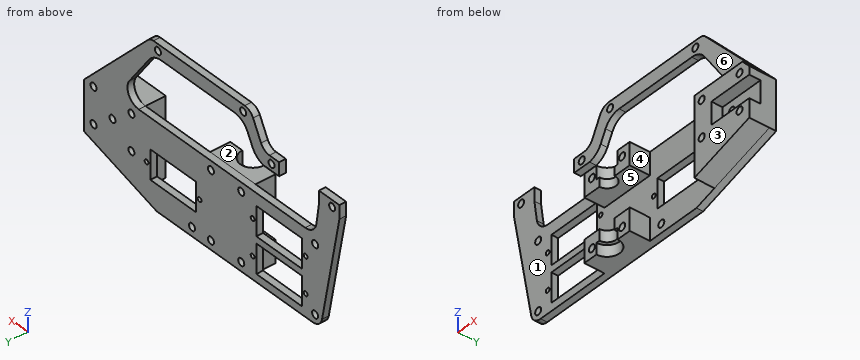
```python
from build123d import *

# Parameters (mm, degrees)
SKETCH_1_R          = 1.6
SKETCH_1_R_2        = 1
SKETCH_1_W          = 24
SKETCH_1_H          = 13
EXTRUDE_1_DEPTH     = 3
SKETCH_2_R          = 1.6
SKETCH_2_W          = 24
SKETCH_2_H          = 10
EXTRUDE_2_DEPTH     = 9
SKETCH_3_W          = 10
SKETCH_3_H          = 10
CUT_EXTRUDE_1_DEPTH = 20
SKETCH_4_R          = 4
CUT_EXTRUDE_2_DEPTH = 72.704206567
SKETCH_6_R          = 5.6
CUT_EXTRUDE_3_DEPTH = 5
SKETCH_7_R          = 5.6
CUT_EXTRUDE_4_DEPTH = 6
FILLET_5_R          = 5
FILLET_6_R          = 5
SKETCH_8_W          = 21
SKETCH_8_H          = 6
CUT_EXTRUDE_5_DEPTH = 13


with BuildPart() as part:
    # Эскиз1 → Бобышка-Вытянуть1 (new body)
    with BuildSketch(Plane(origin=(0, 0, 0), x_dir=(1, 0, 0), z_dir=(0, 1, 0))):
        with BuildLine():
            Line((-59.846473334, -34), (-49.887758312, 18))
            Line((-49.887758312, 18), (36.612736258, 18))
            Line((36.612736258, 18), (75.112241688, 5.920216985))
            Line((75.112241688, 5.920216985), (75.112241688, -16.079783015))
            Line((75.112241688, -16.079783015), (41.245672077, -52.430849732))
            ThreePointArc((41.245672077, -52.430849732), (39.914841322, -53.372078747), (38.318998701, -53.704206567))
            Line((38.318998701, -53.704206567), (-9.799827382, -53.704206567))
            ThreePointArc((-9.799827382, -53.704206567), (-12.412320205, -52.967407389), (-14.254860003, -50.974159066))
            Line((-14.254860003, -50.974159066), (-19.846473334, -40))
            Line((-19.846473334, -40), (-59.846473334, -40))
            Line((-59.846473334, -40), (-59.846473334, -34))
        make_face()
        with Locations((-8, 14)):
            Circle(SKETCH_1_R, mode=Mode.SUBTRACT)
        with Locations((8, 14)):
            Circle(SKETCH_1_R, mode=Mode.SUBTRACT)
        with Locations((-8, -16)):
            Circle(SKETCH_1_R, mode=Mode.SUBTRACT)
        with Locations((8, -16)):
            Circle(SKETCH_1_R, mode=Mode.SUBTRACT)
        with Locations((-47, 14)):
            Circle(SKETCH_1_R, mode=Mode.SUBTRACT)
        with Locations((70, 0)):
            Circle(SKETCH_1_R, mode=Mode.SUBTRACT)
        with Locations((50, 0)):
            Circle(SKETCH_1_R, mode=Mode.SUBTRACT)
        with Locations((18, 14)):
            Circle(SKETCH_1_R, mode=Mode.SUBTRACT)
        with Locations((-47, -16)):
            Circle(SKETCH_1_R, mode=Mode.SUBTRACT)
        with Locations((-56, -37)):
            Circle(SKETCH_1_R, mode=Mode.SUBTRACT)
        with Locations((-24, -37)):
            Circle(SKETCH_1_R, mode=Mode.SUBTRACT)
        with Locations((50, -16)):
            Circle(SKETCH_1_R, mode=Mode.SUBTRACT)
        with Locations((70, -16)):
            Circle(SKETCH_1_R, mode=Mode.SUBTRACT)
        with Locations((-9, -50.704206567)):
            Circle(SKETCH_1_R, mode=Mode.SUBTRACT)
        with Locations((36, -50.704206567)):
            Circle(SKETCH_1_R, mode=Mode.SUBTRACT)
        with Locations((60, -8)):
            Circle(SKETCH_1_R, mode=Mode.SUBTRACT)
        with Locations((-42, -8)):
            Circle(SKETCH_1_R_2, mode=Mode.SUBTRACT)
        with Locations((-14, -8)):
            Circle(SKETCH_1_R_2, mode=Mode.SUBTRACT)
        with Locations((-42, 8)):
            Circle(SKETCH_1_R_2, mode=Mode.SUBTRACT)
        with Locations((-14, 8)):
            Circle(SKETCH_1_R_2, mode=Mode.SUBTRACT)
        with Locations((14, 0)):
            Circle(SKETCH_1_R_2, mode=Mode.SUBTRACT)
        with Locations((42, 0)):
            Circle(SKETCH_1_R_2, mode=Mode.SUBTRACT)
        with Locations((28, 0)):
            Rectangle(SKETCH_1_W, SKETCH_1_H, mode=Mode.SUBTRACT)
        with Locations((-28, 8)):
            Rectangle(SKETCH_1_W, SKETCH_1_H, mode=Mode.SUBTRACT)
        with Locations((-28, -8)):
            Rectangle(SKETCH_1_W, SKETCH_1_H, mode=Mode.SUBTRACT)
        with BuildLine():
            Line((-47.677053254, -24.900709984), (-49.000145857, -34))
            Line((-49.000145857, -34), (-22.297676486, -34))
            Line((-22.297676486, -34), (-19.846473334, -34))
            ThreePointArc((-19.846473334, -34), (-16.425778662, -35.467187694), (-13.988679802, -38.280431537))
            Line((-13.988679802, -38.280431537), (-11.413907263, -43.333707171))
            ThreePointArc((-11.413907263, -43.333707171), (-8.465843587, -46.522904488), (-4.28585507, -47.701783173))
            Line((-4.28585507, -47.701783173), (34.165827616, -47.701783173))
            ThreePointArc((34.165827616, -47.701783173), (37.877016972, -46.788889321), (40.741225842, -44.258551563))
            Line((40.741225842, -44.258551563), (51.02606102, -29.417576293))
            ThreePointArc((51.02606102, -29.417576293), (51.409841961, -23.216607983), (46.09451235, -20))
            Line((46.09451235, -20), (-41.778616049, -20))
            ThreePointArc((-41.778616049, -20), (-45.612951708, -21.385038456), (-47.677053254, -24.900709984))
        make_face(mode=Mode.SUBTRACT)
    extrude(amount=EXTRUDE_1_DEPTH)

    # Эскиз2 → Бобышка-Вытянуть2 (add)
    with BuildSketch(Plane(origin=(0, 0, 0), x_dir=(1, 0, 0), z_dir=(0, 1, 0))):
        Polygon((46.101706289, 15.022696844), (46.09451235, -20), (71.459960933, -20), (75.112241688, -16.079783015), (75.112241688, 5.920216985), align=None)
        with Locations((50, 0)):
            Circle(SKETCH_2_R, mode=Mode.SUBTRACT)
        with Locations((70, 0)):
            Circle(SKETCH_2_R, mode=Mode.SUBTRACT)
        with Locations((70, -16)):
            Circle(SKETCH_2_R, mode=Mode.SUBTRACT)
        with Locations((50, -16)):
            Circle(SKETCH_2_R, mode=Mode.SUBTRACT)
        with Locations((60, -8)):
            Circle(SKETCH_2_R, mode=Mode.SUBTRACT)
        with Locations((0, 13)):
            Rectangle(SKETCH_2_W, SKETCH_2_H)
        with Locations((-8, 14)):
            Circle(SKETCH_2_R, mode=Mode.SUBTRACT)
        with Locations((8, 14)):
            Circle(SKETCH_2_R, mode=Mode.SUBTRACT)
        with Locations((0, -14.961092538)):
            Rectangle(SKETCH_2_W, SKETCH_2_H)
        with Locations((-8, -16)):
            Circle(SKETCH_2_R, mode=Mode.SUBTRACT)
        with Locations((8, -16)):
            Circle(SKETCH_2_R, mode=Mode.SUBTRACT)
    extrude(amount=-EXTRUDE_2_DEPTH)

    # Эскиз3 → Вырез-Вытянуть1 (cut)
    with BuildSketch(Plane(origin=(75.112241688, 0, 0), x_dir=(0, 0, -1), z_dir=(1, 0, 0))):
        with Locations((-7.384625177, -9)):
            Rectangle(SKETCH_3_W, SKETCH_3_H)
    extrude(amount=-CUT_EXTRUDE_1_DEPTH, mode=Mode.SUBTRACT)

    # Эскиз4 → Вырез-Вытянуть2 (cut, through all)
    with BuildSketch(Plane(origin=(0, 0, -18), x_dir=(-1, 0, 0), z_dir=(0, 0, -1))):
        with Locations((0, -9)):
            Circle(SKETCH_4_R)
    extrude(amount=-CUT_EXTRUDE_2_DEPTH, mode=Mode.SUBTRACT)

    # Эскиз6 → Вырез-Вытянуть3 (cut)
    with BuildSketch(Plane(origin=(0, 0, -18), x_dir=(-1, 0, 0), z_dir=(0, 0, -1))):
        with Locations((0, -9)):
            Circle(SKETCH_6_R)
    extrude(amount=-CUT_EXTRUDE_3_DEPTH, mode=Mode.SUBTRACT)

    # Эскиз7 → Вырез-Вытянуть4 (cut)
    with BuildSketch(Plane.XY.offset(19.961092538)):
        with Locations((0, -9)):
            Circle(SKETCH_7_R)
    extrude(amount=-CUT_EXTRUDE_4_DEPTH, mode=Mode.SUBTRACT)

    # Скругление5
    fillet_5_edges = [part.edges().sort_by_distance(p)[0] for p in [
        (-49.887758312, 1.5, -18),
    ]]
    fillet(fillet_5_edges, radius=FILLET_5_R)

    # Скругление6
    fillet_6_edges = [part.edges().sort_by_distance(p)[0] for p in [
        (-19.846473334, 1.5, 40),
    ]]
    fillet(fillet_6_edges, radius=FILLET_6_R)

    # Эскиз8 → Вырез-Вытянуть5 (cut, through all)
    with BuildSketch(Plane(origin=(0, 3, 0), x_dir=(1, 0, 0), z_dir=(0, 1, 0))):
        with Locations((-38.500145857, -37)):
            Rectangle(SKETCH_8_W, SKETCH_8_H)
    extrude(amount=-CUT_EXTRUDE_5_DEPTH, mode=Mode.SUBTRACT)


solid = part.part
```
Could you check a few things on this model? Use its own coordinates, in mm. Face numbers are marked on the shaded views. A direction names the side the tool comes from. Round coordinates to 2 decimals unless told otherwise and drop trailing zeros. Order: outer loops, then holes, each group sorted by start corner. A loop starts at its lowest first (then second) coordinate and runs counter-clockwise, first axis right, second up. Notation, with made-up numbers: (-14, -6) -> (35, -6) arc R26 ccw to (35, 32) -> close; hole circle Ø3 at (51.25, 61). An arc over 180 degrees is marked (long way). One line per question, with ' | ' between items.
Q1. If I drill on line 1 (X direction, y = 0.6, z = 16); line 2 (Z direction, x = 14, y = 1); line 3 (X direction, y = -1, z = 17), over which ranges is the centre line in solid material (lowest first)? Write a range as from..to.
Computed values:
line 1: -56.4..-48.6, -45.4..-9.6, -6.4..6.4, 9.6..48.4, 51.6..68.4, 71.6..75.11 | line 2: -18..-1, 1..20, 47.7..53.7 | line 3: -12..-9.25, -6.75..6.75, 9.25..12, 46.1..48.75, 51.25..68.75, 71.25..74.25
Q2. I'm going to push flat-ended pins straight in: pin 1 (2.5 mm diameter, centred on x = 3.5, y = -5.5, fed in from +Z); pin 2 (4 mm diameter, centred on x = -1.5, z = 12.5, fed in from -Y); pin 3 (1.5 mm diameter, centred on x = -22, y = 1.5, fed in from +Z). Where does each tip first touch, or does it pass through?
Computed values:
pin 1: z = 19.96 | pin 2: y = -7.06 | pin 3: z = 40.28
Q3. If we section it at C-C on x = -38: Write out the boundary of the cut face in (y, z), plus the area to 3 significant figures.
Computed values:
outline: (0, -18) -> (3, -18) -> (3, -14.5) -> (0, -14.5) -> close; (0, -1.5) -> (3, -1.5) -> (3, 1.5) -> (0, 1.5) -> close; (0, 14.5) -> (3, 14.5) -> (3, 20) -> (0, 20) -> close | area: 36.0 mm²
Q4. Which directions (+Z, -Z, +X, -X, +Y, -Y) give clear straight access to the entire face, cutting with the end or side of a thin tool? Please do the marked faces 4, 5 and 6.
Computed values:
face 4: +Z, -Z, -Y | face 5: -X, -Y | face 6: +Z, +X, -X, -Y
Q5. If we section it at D-D on x = 18: Write out the boundary of the cut face in (y, z), plus the area to 3 significant figures.
Computed values:
outline: (0, -18) -> (3, -18) -> (3, -15.6) -> (0, -15.6) -> close; (0, -12.4) -> (3, -12.4) -> (3, -6.5) -> (0, -6.5) -> close; (0, 6.5) -> (3, 6.5) -> (3, 20) -> (0, 20) -> close; (0, 47.7) -> (3, 47.7) -> (3, 53.7) -> (0, 53.7) -> close | area: 83.4 mm²
Q6. We'd pull the mould along Z, two halves only. Please class the marked faces 1, 2 and 3: released by +Z, released by -Z, zero draft, split by the parting line, or undercut.
Computed values:
face 1: undercut | face 2: released by +Z | face 3: zero draft
Q7. If we section it at B-B on z = -11: Write out the boundary of the cut face in (x, y).
Computed values:
outline: (-51.23, 0) -> (-40, 0) -> (-40, 3) -> (-51.23, 3) -> close; (-16, 0) -> (-12, 0) -> (-12, -9) -> (-4, -9) arc R4 cw to (4, -9) -> (12, -9) -> (12, 0) -> (46.1, 0) -> (46.1, -9) -> (58.92, -9) -> (58.92, 3) -> (-16, 3) -> close
